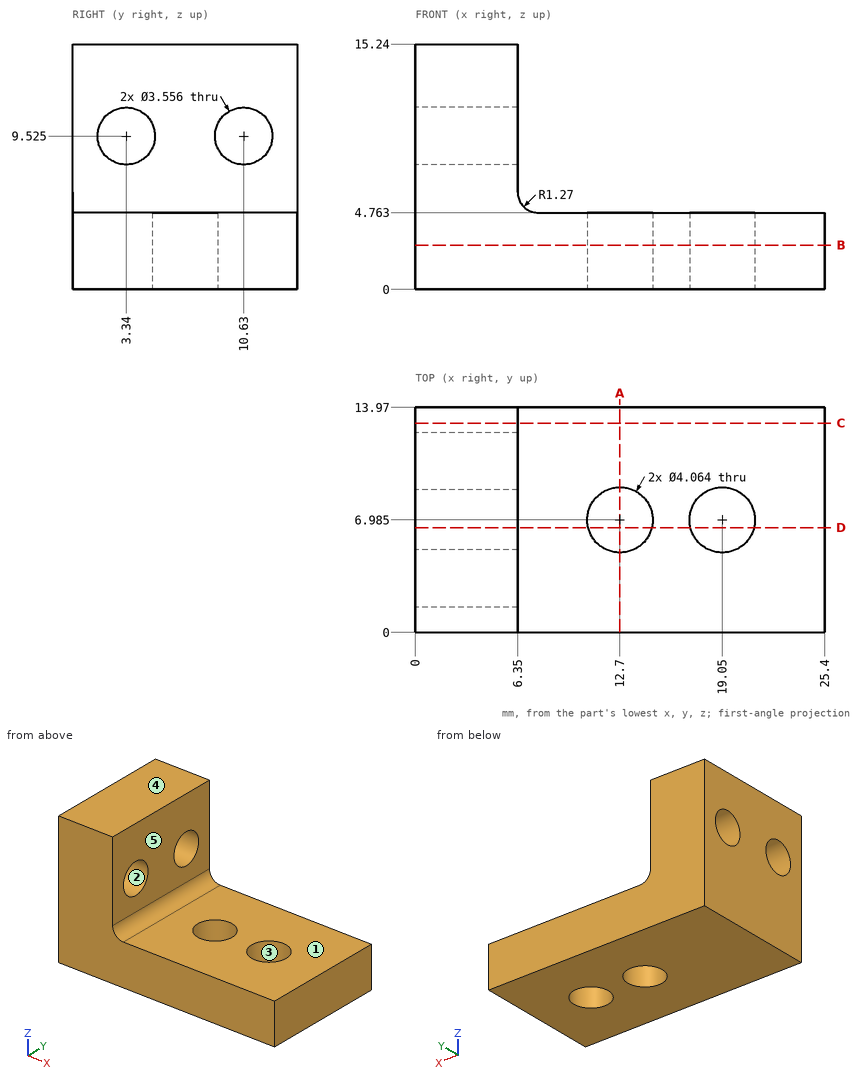
For this review, use the dimensioned drawing (mm, ordinates from the lowest corner) and the shaded views. A direction names the side the tool comes from. Coordinates: 2 decimals unless noted, no trailing zeros. Loops run counter-clockwise (first coordinate to the right, second up) from the corner with the lowest first, then second, coordinate; pieces in that order, holes last. Notation, with made-up numbers: (-31, 16.25) - (13, 16.25) arc R23 ccw to (13, 24.25) - close; hole circle Ø7 at (21, 14.5). An arc over 180 degrees is marked (long way). Use one line per item in the form item = value. Start each with the question number.
1) Take a section at D-D (y = 6.5). State the section outline as (x, z) points.
2) For pin 1 (4.5 mm diameter, centred on y = 8, z = 9.5, fed in from +X); pin 2 (3.5 mm diameter, centred on x = 19.05, y = 6.985, fed in from +Z); pin 3 (1.5 mm diameter, centred on x = 11.5, y = 2, fed in from +Z), all flat-tipped, find the tip position at first contact; note any pin that passes through.
3) Draft analysis for pull direction Z (two halves, no side actions). For the marked faces 1, 2 and 3, state which applies: released by +Z, released by -Z, zero draft, split by the parting line, or undercut.
4) To check wall thickness, follow probe 1 along X at (y, z) = (7.25, 4) (1 decimal); probe 2 along X at (y, z) = (6.25, 4.25) (1 decimal); probe 3 along Y at (x, z) = (12.7, 2.95). State the ranges of each line that lie inside material, in increasing order. Write a range as from..to.
5) Take a section at C-C (y = 13). State the section outline as (x, z) points.
6) Take a section at A-A (x = 12.7). State the section outline as (y, z) points.
7) For the marked faces 4 and 5, list the 3-axis set-ups (+Z, -Z, +X, -X, +Y, -Y) from which the entire face can be reached by the end or side of a thin tool; tool diameter is ignored.
8) Take a section at B-B (z = 2.75). State how many separate pieces and enclosed holes the cut face has, plus the area to 3 significant figures.
From the geometry:
q1.outline = (0, 0) - (10.73, 0) - (10.73, 4.76) - (7.62, 4.76) arc R1.27 cw to (6.35, 6.03) - (6.35, 15.24) - (0, 15.24) - close; (14.67, 0) - (17.08, 0) - (17.08, 4.76) - (14.67, 4.76) - close; (21.02, 0) - (25.4, 0) - (25.4, 4.76) - (21.02, 4.76) - close
q2.pin_1 = 6.35
q2.pin_2 = through
q2.pin_3 = 4.76
q3.face_1 = released by +Z
q3.face_2 = undercut
q3.face_3 = zero draft
q4.probe_1 = 0..10.7, 14.7..17, 21.1..25.4
q4.probe_2 = 0..10.8, 14.6..17.2, 20.9..25.4
q4.probe_3 = 0..4.95, 9.02..13.97
q5.outline = (0, 0) - (25.4, 0) - (25.4, 4.76) - (7.62, 4.76) arc R1.27 cw to (6.35, 6.03) - (6.35, 15.24) - (0, 15.24) - close
q6.outline = (0, 0) - (4.95, 0) - (4.95, 4.76) - (0, 4.76) - close; (9.02, 0) - (13.97, 0) - (13.97, 4.76) - (9.02, 4.76) - close
q7.face_4 = +Z, +X, -X, +Y, -Y
q7.face_5 = +Z, +X, +Y, -Y
q8.separate_pieces = 1
q8.enclosed_holes = 2
q8.area = 329 mm2
